from build123d import *

# Parameters (mm, degrees)
BOSS_EXTRUDE1_DEPTH = 635


with BuildPart() as part:
    # Sketch3 → Boss-Extrude1 (new body)
    with BuildSketch(Plane.XY):
        with BuildLine():
            Line((-2079.212661728, -769.863228), (-860.012661728, -769.863228))
            ThreePointArc((-860.012661728, -769.863228), (-770.210100518, -732.665789211), (-733.012661728, -642.863228))
            Line((-733.012661728, -642.863228), (-733.012661728, 246.136772))
            Line((-733.012661728, 246.136772), (-428.150553924, 246.136772))
            Line((-428.150553924, 246.136772), (-428.150553924, -7.863228))
            Line((-428.150553924, -7.863228), (-326.612661728, -7.863228))
            Line((-326.612661728, -7.863228), (-318.929679791, -7.863228))
            Line((-318.929679791, -7.863228), (-318.929679791, -84.063228))
            ThreePointArc((-318.929679791, -84.063228), (-157.578570713, -360.389072068), (143.287338272, -469.33794683))
            Line((143.287338272, -469.33794683), (143.287338272, -896.863228))
            Line((143.287338272, -896.863228), (-2079.212661728, -896.863228))
            Line((-2079.212661728, -896.863228), (-2079.212661728, -769.863228))
        make_face()
    extrude(amount=BOSS_EXTRUDE1_DEPTH)


solid = part.part
Could you check a few things on this model? Use its own coordinates, in mm. A direction names the side the tool comes from. Coordinates: 2 decimals unless noted, no trailing zeros. Loops run counter-clockwise (first coordinate to the right, second up) from the corner with the lowest first, then second, coordinate; pieces in that order, holes last.
1. I need wall thicknesses on L1, parallel to X at y = -540, z = 531; L2, parallel to X at y = 2, z = 182; L3, parallel to Y at x = -1127.5, z = 273. Which ranges of each line are inside material? Lowest first, please.
2. For faces 1 (the face through (-318.93, -45, 313)), 2 (the face through (-733.013, -205, 313)), 3 (the face through (-705, -444, 635)), which set-ups out of +Z, -Z, +X, -X, +Y, -Y let a thin tool reach every point of the face, with its end or its side?
3. For P1, Ø6, axis at y = -466, z = 439.5, coming from the -X side, with a flat end and sliding along its axis, tell me the tip position at first contact or that it passes through.
4. Imagine slicing it at C-C (y = -502.5). Please give me the cut outline in (x, z).
5. Imagine slicing it at B-B (x = -388). Please give me the cut outline in (y, z).
6. Imagine slicing it at A-A (z = 458). Please give me the cut outline in (x, y), and give its area (3 significant figures).
Computed values:
1. L1: x = -733.01 to 143.29
1. L2: x = -733.01 to -428.15
1. L3: y = -896.86 to -769.86
2. face 1: +Z, -Z, +X, +Y
2. face 2: +Z, -Z, -X, +Y
2. face 3: +Z, +X, -X, +Y, -Y
3. P1: stops at x = -733.01
4. outline: (-733.01, 0) - (143.29, 0) - (143.29, 635) - (-733.01, 635) - close
5. outline: (-896.86, 0) - (-7.86, 0) - (-7.86, 635) - (-896.86, 635) - close
6. outline: (-2079.21, -896.86) - (143.29, -896.86) - (143.29, -469.34) arc R469.9 cw to (-318.93, -84.06) - (-318.93, -7.86) - (-428.15, -7.86) - (-428.15, 246.14) - (-733.01, 246.14) - (-733.01, -642.86) arc R127 cw to (-860.01, -769.86) - (-2079.21, -769.86) - close
6. area: 862,000 mm2
